```python
from build123d import *

# Parameters (mm, degrees)
F0_R     = 11.075
F1_DEPTH = 3.6


# Not quite as in the source:
# - a feature of the source that left no trace in its solid (it failed there, or was rolled back) is left out


with BuildPart() as f1:
    # F0 (on Front) → F1 (new body, symmetric)
    with BuildSketch(Plane.XZ):
        with BuildLine():
            Line((-18.7389361234, 0.3405199539), (-14.7669712633, 2.6337349351))
            ThreePointArc((-14.7669712633, 2.6337349351), (-11.8584662517, -9.1856833256), (-1.1413957778, -14.9565108123))
            Line((-1.1413957778, -14.9565108123), (1.2456877462, -17.2733709451))
            Line((1.2456877462, -17.2733709451), (-5.4411288371, -21.6098797995))
            ThreePointArc((-5.4411288371, -21.6098797995), (-0.2713631395, -39.9963174243), (5.8883015494, -21.9174320378))
            Line((5.8883015494, -21.9174320378), (9.0745691311, -16.3986546997))
            Line((9.0745691311, -16.3986546997), (5.102604271, -14.1054397185))
            ThreePointArc((5.102604271, -14.1054397185), (13.8842682369, -5.6768913611), (13.5234162043, 6.4897776668))
            Line((13.5234162043, 6.4897776668), (14.3363341744, 9.7154827059))
            Line((14.3363341744, 9.7154827059), (21.4352692976, 6.0927841016))
            ThreePointArc((21.4352692976, 6.0927841016), (34.773508517, 19.7631513397), (16.0369021558, 16.0581347458))
            Line((16.0369021558, 16.0581347458), (9.6643669923, 16.0581347458))
            Line((9.6643669923, 16.0581347458), (9.6643669923, 11.4717047835))
            ThreePointArc((9.6643669923, 11.4717047835), (-2.0258019852, 14.8625746867), (-12.3820204265, 8.4667331455))
            Line((-12.3820204265, 8.4667331455), (-15.5820219205, 7.5578882392))
            Line((-15.5820219205, 7.5578882392), (-15.9941404606, 15.5170956979))
            ThreePointArc((-15.9941404606, 15.5170956979), (-34.5021453775, 20.2331660846), (-21.9252037051, 5.859297292))
            Line((-21.9252037051, 5.859297292), (-18.7389361234, 0.3405199539))
        make_face()
        Polygon((0, -22.4944465005), (6.5, -26.2472232503), (6.5, -33.7527767497), (0, -37.5055534995), (-6.5, -33.7527767497), (-6.5, -26.2472232503), align=None, mode=Mode.SUBTRACT)
        Circle(F0_R, mode=Mode.SUBTRACT)
        Polygon((-32.4807621135, 11.2472232503), (-32.4807621135, 18.7527767497), (-25.9807621135, 22.5055534995), (-19.4807621135, 18.7527767497), (-19.4807621135, 11.2472232503), (-25.9807621135, 7.4944465005), align=None, mode=Mode.SUBTRACT)
        Polygon((25.9807621135, 22.5055534995), (32.4807621135, 18.7527767497), (32.4807621135, 11.2472232503), (25.9807621135, 7.4944465005), (19.4807621135, 11.2472232503), (19.4807621135, 18.7527767497), align=None, mode=Mode.SUBTRACT)
    extrude(amount=F1_DEPTH, both=True)


solid = f1.part
```
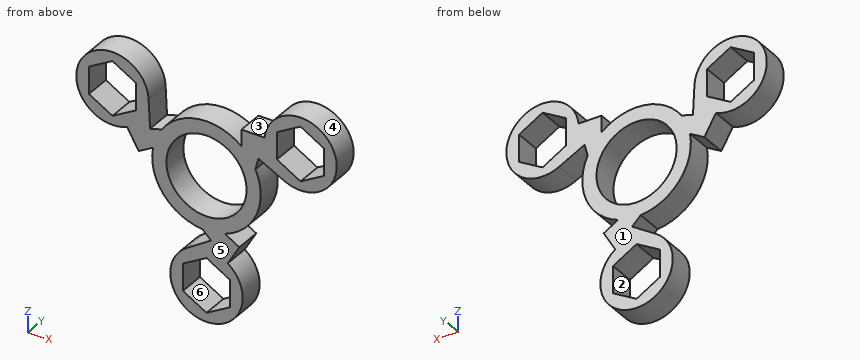
For this review, take the finished solid that the model builds, in its own axes (mm). Face numbers are marked on the shaded views. A direction names the side the tool comes from. Round coordinates to 2 decimals unless told otherwise and drop trailing zeros. Write each loop counter-clockwise with the first axis right and the second up, starting at its lowest first coordinate (ties: lowest second). Pieces come first, ordered by that corner, then holes.
1) Take a section at A-A on z = -30. Give the boundary of the cut face in (x, y).
Answer below:
outline: (-10, -3.6) - (-6.5, -3.6) - (-6.5, 3.6) - (-10, 3.6) - close; (6.5, -3.6) - (10, -3.6) - (10, 3.6) - (6.5, 3.6) - close
2) Insertion check: pin 1 Ø1.9 at (x, y) = (14, 0) entering from +Z; pin 2 Ø1.5 at (x, y) = (-4, -1.5) entering from +Z; pin 3 Ø2 at (y, z) = (0.5, -16) entering from +X. Each pin has a flat end and moves straight along its axis. Give the tip position at first contact, or say it passes through.
Answer below:
pin 1: stops at z = 16.06
pin 2: stops at z = 14.64
pin 3: stops at x = 9.07
3) Take a section at C-C on z = 13.5. Give the boundary of the cut face in (x, y).
Answer below:
outline: (-35.87, -3.6) - (-32.48, -3.6) - (-32.48, 3.6) - (-35.87, 3.6) - close; (-19.48, -3.6) - (-15.89, -3.6) - (-15.89, 3.6) - (-19.48, 3.6) - close; (-6.54, -3.6) - (6.54, -3.6) - (6.54, 3.6) - (-6.54, 3.6) - close; (9.66, -3.6) - (19.48, -3.6) - (19.48, 3.6) - (9.66, 3.6) - close; (32.48, -3.6) - (35.87, -3.6) - (35.87, 3.6) - (32.48, 3.6) - close
4) Take a section at B-B on x = 24. Give the boundary of the cut face in (y, z).
Answer below:
outline: (-3.6, 5.2) - (3.6, 5.2) - (3.6, 8.64) - (-3.6, 8.64) - close; (-3.6, 21.36) - (3.6, 21.36) - (3.6, 24.8) - (-3.6, 24.8) - close
5) For line 1 along Z through (x, y) = (3, 1.5); line 2 along X through (y, z) = (-2.25, 21); line 3 along X through (y, z) = (1.75, 2), list the stretches that pass through material, from the lowest coordinate up.
Answer below:
line 1: z = -39.54 to -35.77, -24.23 to -10.66, 10.66 to 14.7
line 2: x = -33.98 to -28.59, -23.37 to -17.98, 17.98 to 23.37, 28.59 to 33.98
line 3: x = -19.7 to -15.86, -14.87 to -10.89, 10.89 to 14.87
6) Machinability: for the marked faces 1, 2 and 3, which of the approach directions +Z, -Z, +X, -X, +Y, -Y give a long, thin tool a straight path to every point of the face, cutting with its end or side? Answer none if there is none.
Answer below:
face 1: +Z, -Z, +X, -X, +Y
face 2: +Y, -Y
face 3: +Z, +Y, -Y
7) Mouldability with a two-part tool opening along Z and no side actions: class the marked faces 4, 5 and 6 as +Z half, -Z half, draft (parallel to the pull), parting line (faces both ways), or undercut.
Answer below:
face 4: parting line
face 5: draft
face 6: undercut
8) Take a section at D-D on x = -7.5. Give the boundary of the cut face in (y, z), then the cut area to 3 significant figures.
Answer below:
outline: (-3.6, -36.61) - (3.6, -36.61) - (3.6, -23.39) - (-3.6, -23.39) - close; (-3.6, -12.99) - (3.6, -12.99) - (3.6, -8.15) - (-3.6, -8.15) - close; (-3.6, 8.15) - (3.6, 8.15) - (3.6, 12.99) - (-3.6, 12.99) - close
area: 165 mm2
